from build123d import *

# Parameters (mm, degrees)
SKETCH1_R           = 6.35
BOSS_EXTRUDE1_DEPTH = 12.7


with BuildPart() as part:
    # Sketch1 → Boss-Extrude1 (new body)
    with BuildSketch(Plane.XY):
        with BuildLine():
            Line((-120.015, 12.7), (-31.809733165, 12.7))
            ThreePointArc((-31.809733165, 12.7), (-22.808332465, 16.416135762), (-19.05, 25.4))
            ThreePointArc((-19.05, 25.4), (0, 44.45), (19.05, 25.4))
            ThreePointArc((19.05, 25.4), (22.808332465, 16.416135762), (31.809733165, 12.7))
            Line((31.809733165, 12.7), (120.015, 12.7))
            ThreePointArc((120.015, 12.7), (132.715, 0), (120.015, -12.7))
            Line((120.015, -12.7), (-120.015, -12.7))
            ThreePointArc((-120.015, -12.7), (-132.715, 0), (-120.015, 12.7))
        make_face()
        with Locations((-120.015, 0)):
            Circle(SKETCH1_R, mode=Mode.SUBTRACT)
        with Locations((120.015, 0)):
            Circle(SKETCH1_R, mode=Mode.SUBTRACT)
        with Locations((0, 25.4)):
            Circle(SKETCH1_R, mode=Mode.SUBTRACT)
    extrude(amount=BOSS_EXTRUDE1_DEPTH)


solid = part.part
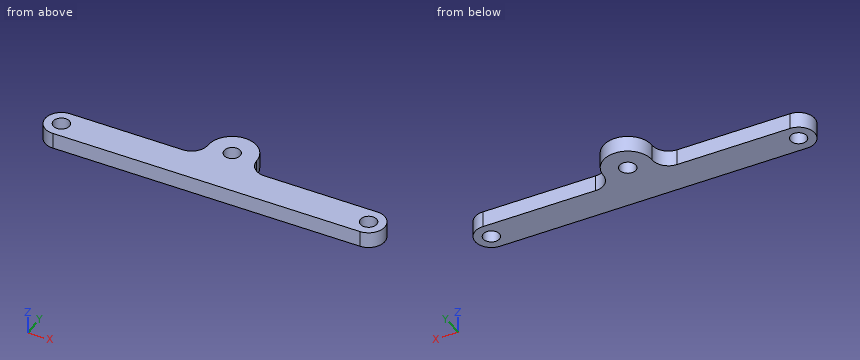
Model file for the job. Use its own axes, mm. Give positions to 0.01 mm unless a question says otherwise; leave off trailing zeros. Loops run counter-clockwise (first coordinate to the right, second up) from the corner with the lowest first, then second, coordinate; pieces in that order, holes last.
1) Saw through at C-C (z = 9.25). Write the cut outline in (x, y) (3 decimals).
2) Saw through at A-A (y = 0). Write the cut outline in (x, z) (3 decimals).
3) Wall check: line 1 (X direction, y = -4, z = 9.5); line 2 (X direction, y = -3, z = 5.5); line 3 (Y direction, x = 0, z = 6). Give the ranges that are in metal, low to high.
4) Saw through at D-D (y = 40). Write the cut outline in (x, z), plus the area to 3 significant figures.
5) Flat gauge pins, fed straight in: pin 1 Ø3 at (x, z) = (-38.5, 6.5) entering from +Y; pin 2 Ø1 at (x, y) = (47.5, 14) entering from +Z; pin 3 Ø3 at (y, z) = (10.5, 10) entering from +X; pin 4 Ø2 at (y, z) = (28, 8.5) entering from -X. Where does each tip first touch, or does it go through?
6) Saw through at B-B (x = 0). Write the cut outline in (y, z).
Answer block:
1. outline: (-120.015, -12.7) - (120.015, -12.7) arc R12.7 ccw to (120.015, 12.7) - (31.81, 12.7) arc R12.76 cw to (19.05, 25.4) arc R19.05 ccw to (-19.05, 25.4) arc R12.76 cw to (-31.81, 12.7) - (-120.015, 12.7) arc R12.7 ccw to start; hole circle Ø12.7 at (-120.015, 0); hole circle Ø12.7 at (0, 25.4); hole circle Ø12.7 at (120.015, 0)
2. outline: (-132.715, 0) - (-126.365, 0) - (-126.365, 12.7) - (-132.715, 12.7) - close; (-113.665, 0) - (113.665, 0) - (113.665, 12.7) - (-113.665, 12.7) - close; (126.365, 0) - (132.715, 0) - (132.715, 12.7) - (126.365, 12.7) - close
3. line 1: x = -132.07 to -124.95, -115.08 to 115.08, 124.95 to 132.07
3. line 2: x = -132.36 to -125.61, -114.42 to 114.42, 125.61 to 132.36
3. line 3: y = -12.7 to 19.05, 31.75 to 44.45
4. outline: (-12.24, 0) - (12.24, 0) - (12.24, 12.7) - (-12.24, 12.7) - close
4. area: 311 mm2
5. pin 1: stops at y = 12.7
5. pin 2: passes through
5. pin 3: stops at x = 128.98
5. pin 4: stops at x = -18.98
6. outline: (-12.7, 0) - (19.05, 0) - (19.05, 12.7) - (-12.7, 12.7) - close; (31.75, 0) - (44.45, 0) - (44.45, 12.7) - (31.75, 12.7) - close
